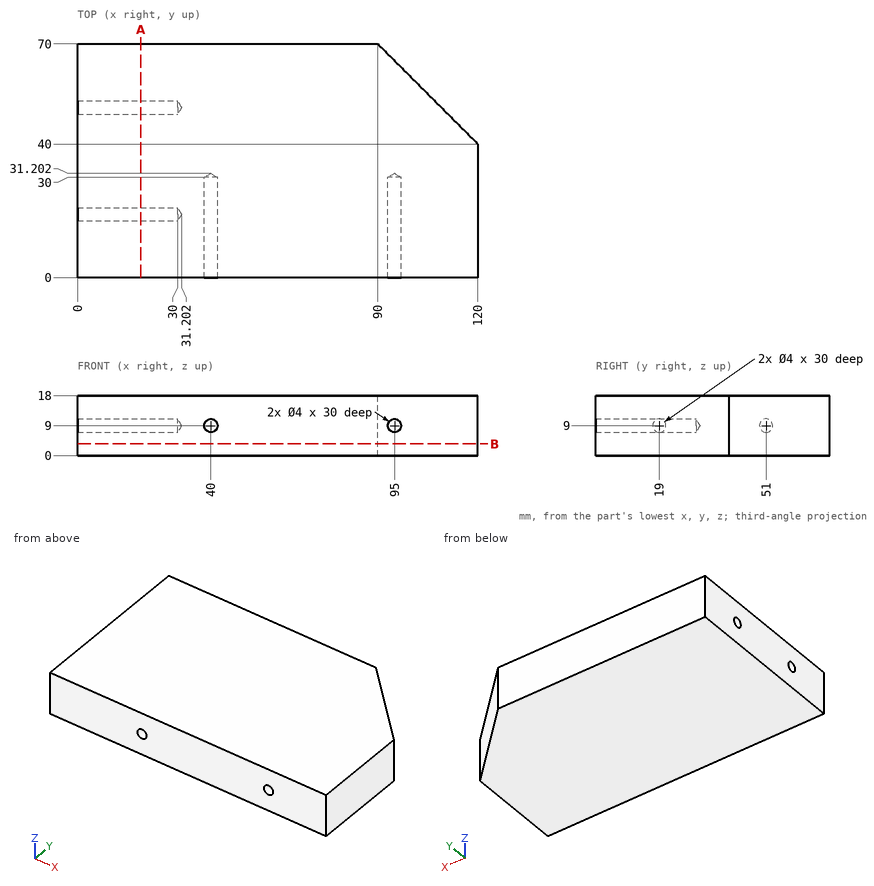
Check sheet for the drawn part. Datum: minimum x, y, z corner. Units: mm. Give positions to 0.01 mm unless a question says otherwise; leave off trailing zeros. Order: outer loops, then holes, each group sorted by start corner. A loop starts at its lowest first (then second) coordinate and runs counter-clockwise, first axis right, second up. Notation, with made-up numbers: (70.5, 57.25) -> (127.5, 57.25) arc R17 ccw to (127.5, 68.25) -> close; hole circle Ø1 at (49, 48). An arc over 180 degrees is marked (long way). One line per item, written item: value.
(1) Sectioned sample at B-B on z = 3.5. Record the cut outline in (x, y).
Final values:
outline: (0, 0) -> (120, 0) -> (120, 40) -> (90, 70) -> (0, 70) -> close
(2) Sectioned sample at A-A on x = 19. Record the cut outline in (y, z), then the cut area to 3 significant figures.
Final values:
outline: (0, 0) -> (70, 0) -> (70, 18) -> (0, 18) -> close; hole circle Ø4 at (19, 9); hole circle Ø4 at (51, 9)
area: 1,230 mm^2
(3) Gauge pin test, flat ends, axial feed: pin 1 (10 mm diameter, centred on y = 35.5, z = 3.5, fed in from -X); pin 2 (1.5 mm diameter, centred on y = 61, z = 5.5, fed in from +X); pin 3 (2.5 mm diameter, centred on x = 95, z = 9, fed in from +Y). Record the tip position at first contact, or that the pin passes through.
Final values:
pin 1: x = 0
pin 2: x = 99.75
pin 3: y = 66.25
(4) Scan lines: line 1 along X through (y, z) = (12.5, 9); line 2 along Z through (x, y) = (40, 15.25); line 3 along X through (y, z) = (20.5, 7.25). Record each from-to range of solid material in increasing order. Write a range as [from, to].
Final values:
line 1: [0, 38], [42, 93], [97, 120]
line 2: [0, 7], [11, 18]
line 3: [0, 39.03], [40.97, 94.03], [95.97, 120]
